from build123d import *

# Parameters (mm, degrees)
PAD001_DEPTH           = 10
PAD002_DEPTH           = 15
FILLET_R               = 3.3
SKETCH007_R            = 10.5
SKETCH007_R_2          = 4.5
POCKET001_DEPTH        = 7
LINEARPATTERN001_COUNT = 3
LINEARPATTERN001_PITCH = 35
SKETCH008_W            = 20
SKETCH008_H            = 0.204143
PAD004_DEPTH           = 38
SKETCH009_R            = 4
PAD005_DEPTH           = 14
SKETCH010_R            = 4
PAD006_DEPTH           = 11


with BuildPart() as part:
    # Sketch001 → Pad001 (new body)
    with BuildSketch(Plane.XY):
        with BuildLine():
            add(Edge.make_bspline(
                [(-21, 0), (-21, -130), (0, -130), (21, -130), (21, 0)],
                knots=[4.712389, 4.712389, 4.712389, 6.283185, 6.283185, 7.853982, 7.853982, 7.853982], degree=2, weights=[1, 0.707107, 1, 0.707107, 1]))
            Line((21, 0), (-21, 0))
        make_face()
    extrude(amount=-PAD001_DEPTH)

    # Sketch004 (on Face4 of Pad001) → Pad002 (join)
    with BuildSketch(Plane(origin=(0, 0, 0), x_dir=(1, 0, 0), z_dir=(0, 0, -1))):
        with BuildLine():
            add(Edge.make_bspline(
                [(14.127174, 100.12989), (0, 172.550511), (-14.127174, 100.12989)],
                knots=[2.356331, 2.356331, 2.356331, 3.926854, 3.926854, 3.926854], degree=2, weights=[1, 0.707203, 1]))
            Line((-14.127174, 100.12989), (14.127174, 100.12989))
        make_face()
    extrude(amount=PAD002_DEPTH)

    # Fillet
    fillet_edges = [part.edges().sort_by_distance(p)[0] for p in [
        (-0.005047, -130.129887, -15),
        (0, -100.12989, -15),
        (19.368374, -50.240623, -10),
        (-19.368374, -50.240623, -10),
    ]]
    fillet(fillet_edges, radius=FILLET_R)

    # Sketch007 → Pocket001 (cut)
    with BuildSketch(Plane.XY):
        with Locations((0, -90)):
            Circle(SKETCH007_R)
        with Locations((0, -90)):
            Circle(SKETCH007_R_2, mode=Mode.SUBTRACT)
    pocket001 = extrude(amount=-POCKET001_DEPTH, mode=Mode.SUBTRACT)

    # LinearPattern001: Pocket001 ×3
    with Locations(*[(0, i * LINEARPATTERN001_PITCH, 0) for i in range(1, LINEARPATTERN001_COUNT)]):
        add(pocket001, mode=Mode.SUBTRACT)

    # Sketch008 (on Face5 of LinearPattern001) → Pad004 (join)
    with BuildSketch(Plane(origin=(0, 0, 0), x_dir=(-1, 0, 0), z_dir=(0, 1, 0))):
        with Locations((7.869961, -9.70371)):
            Rectangle(SKETCH008_W, SKETCH008_H)
    extrude(amount=PAD004_DEPTH)

    # Sketch009 (on Face16 of Pad004) → Pad005 (join)
    with BuildSketch(Plane.XY.offset(-9.601639)):
        with Locations((0, 13)):
            Circle(SKETCH009_R)
    extrude(amount=PAD005_DEPTH)

    # Sketch010 (on Face16 of Pad005) → Pad006 (join)
    with BuildSketch(Plane.XY.offset(-9.601639)):
        with Locations((-8, 32)):
            Circle(SKETCH010_R)
    extrude(amount=PAD006_DEPTH)


solid = part.part
Geometry check sheet. Reference: the model listing, model coordinates, mm. A direction names the side the tool comes from. Round coordinates to 2 decimals unless told otherwise and drop trailing zeros. Loops run counter-clockwise (first coordinate to the right, second up) from the corner with the lowest first, then second, coordinate; pieces in that order, holes last.
Item 1: Cross-section at B-B on y = 32. Record the boundary of the cut face in (x, z).
Item 2: Cross-section at A-A on z = -3.25. Count the separate pieces of the cut face and the enclosed holes in it, then the cut area to 3 significant figures.
Item 3: Access from +Z, -Z, +X, -X, +Y, -Y to the whole of each face (thin tool, end or side, straight path). Record for faces 5 (the flat face through (-8, 19, -9.806)), 6 (the flat face through (0, -90, 0)), 7 (the cylindrical face through (-0.59, -85.54, -3.45)).
Item 4: Mould release check, pull along Y, two halves, no side actions. Record for faces 1 (the cylindrical face through (0.198, -101.071, -14.008)), 2 (the flat face through (0, -49, -10)), 3 (the cylindrical face through (10, -16.8, -3.5)), 4 (the cylindrical face through (2.08, -58.99, -3.45)): pulls with the +Y half, pulls with the -Y half, needs draft (parallel to the pull), parting line crosses it, or undercut.
Item 5: Gauge pin test, flat ends, axial feed: pin 1 (3 mm diameter, centred on x = 15.5, y = -51, fed in from -Z); pin 2 (3 mm diameter, centred on x = -1.5, y = -76, fed in from +Z); pin 3 (16 mm diameter, centred on x = -12, y = 21, fed in from +Z). Record the tip position at first contact, or that the pin passes through.
Item 6: Thickness scan on line 1 (Z direction, x = -17.5, y = -54); line 2 (X direction, y = -3, z = -5.25); line 3 (Z direction, x = -4, y = -13.5). Record the ranges inside material, lowest first.
Answer sheet:
1. outline: (-17.87, -9.81) - (2.13, -9.81) - (2.13, -9.6) - (-4, -9.6) - (-4, 1.4) - (-12, 1.4) - (-12, -9.6) - (-17.87, -9.6) - close
2. separate pieces: 6
2. enclosed holes: 3
2. area: 3,580 mm2
3. face 5: -Z, +X, -X, +Y
3. face 6: +Z, +X, -X, -Y
3. face 7: +Z
4. face 1: pulls with the +Y half
4. face 2: needs draft
4. face 3: undercut
4. face 4: undercut
5. pin 1: stops at z = -10
5. pin 2: stops at z = 0
5. pin 3: stops at z = 1.4
6. line 1: z = -9.53 to 0
6. line 2: x = -20.99 to 20.99
6. line 3: z = -10 to -7
